Could you check a few things on this model? Use its own coordinates, in mm. A direction names the side the tool comes from. Give positions to 0.01 mm unless a question says otherwise; leave off trailing zeros. Loops run counter-clockwise (first coordinate to the right, second up) from the corner with the lowest first, then second, coordinate; pieces in that order, holes last. Notation, with made-up numbers: M 50,74.5 L 92,74.5 A18 ccw 92,91.5 Z; hole C 45.25,-38.75 d8. An arc over 180 degrees is marked long. Use CSV: the item, a comma, the result in double quotes.
```python
from build123d import *

# Parameters (mm, degrees)
SKETCH3_R           = 3.3
SKETCH3_R_2         = 2.3
BOSS_EXTRUDE3_DEPTH = 7
SKETCH4_R           = 5
SKETCH4_R_2         = 3.3
BOSS_EXTRUDE4_DEPTH = 2
SKETCH5_R           = 2.3
SKETCH5_R_2         = 1.7
BOSS_EXTRUDE5_DEPTH = 1


with BuildPart() as part:
    # Sketch3 → Boss-Extrude3 (new body)
    with BuildSketch(Plane(origin=(0, 0, 0), x_dir=(1, 0, 0), z_dir=(0, 1, 0))):
        Circle(SKETCH3_R)
        Circle(SKETCH3_R_2, mode=Mode.SUBTRACT)
    extrude(amount=BOSS_EXTRUDE3_DEPTH)

    # Sketch4 → Boss-Extrude4 (add)
    with BuildSketch(Plane.XZ):
        Circle(SKETCH4_R)
        Circle(SKETCH4_R_2, mode=Mode.SUBTRACT)
    extrude(amount=-BOSS_EXTRUDE4_DEPTH)

    # Sketch5 → Boss-Extrude5 (add)
    with BuildSketch(Plane(origin=(0, 7, 0), x_dir=(1, 0, 0), z_dir=(0, 1, 0))):
        Circle(SKETCH5_R)
        Circle(SKETCH5_R_2, mode=Mode.SUBTRACT)
    extrude(amount=-BOSS_EXTRUDE5_DEPTH)


solid = part.part
```
1. I'm going to push flat-ended pins straight in: pin 1 Ø4 at (y, z) = (1.5, 4) entering from -X; pin 2 Ø2 at (x, y) = (-3, 2.5) entering from -Z; pin 3 Ø1 at (x, y) = (-0.5, 3) entering from -Z. Where does each tip first touch, or does it pass through?
Outcome:
pin 1,"x = -4.58"
pin 2,"z = -4.52"
pin 3,"z = -3.3"
2. I want a section at D-D, the plane x = -4. List the corners of the cut face in (y, z) for me, then the cut area to 3 significant figures.
Outcome:
outline,"M 0,-3 L 2,-3 L 2,3 L 0,3 Z"
area,"12.0 mm2"
3. Which directions (+Z, -Z, +X, -X, +Y, -Y) give clear straight access to the entire face, cutting with the end or side of a thin tool? Please do faces 1 (the face through (-1.08, 0.99, -4.88)), 2 (the face through (-1.825, 2.958, 1.4)).
Outcome:
face 1,"+Y, -Y"
face 2,"-Y"
4. I want a section at C-C, the plane y = 4. List the corners of the cut face in (x, z) for me, then the cut area to 3 significant figures.
Outcome:
outline,"C 0,0 d6.6; hole C 0,0 d4.6"
area,"17.6 mm2"
5. Please list where these lines run through material, in increasing order: line 1 (X direction, y = 6.6, z = 0); line 2 (X direction, y = 3, z = 0).
Outcome:
line 1,"-3.3 to -1.7, 1.7 to 3.3"
line 2,"-3.3 to -2.3, 2.3 to 3.3"
6. If we mould it in two halves opening along Z, with no side actions, what happens to faces 3 (the face through (-0.37, 6.51, 1.66)), 4 (the face through (-2.43, 4.46, -2.23)), 5 (the face through (-1.2, 2, -3.3))? For each: +Z half, -Z half, draft (parallel to the pull), parting line (faces both ways), or undercut.
Outcome:
face 3,"undercut"
face 4,"parting line"
face 5,"draft"
7. I want a section at B-B, the plane x = -1.5. List the corners of the cut face in (y, z) for me, then the cut area to 4 significant figures.
Outcome:
outline,"M 0,-4.77 L 2,-4.77 L 2,-2.94 L 7,-2.94 L 7,-0.8 L 6,-0.8 L 6,-1.74 L 0,-1.74 Z; M 0,1.74 L 6,1.74 L 6,0.8 L 7,0.8 L 7,2.94 L 2,2.94 L 2,4.77 L 0,4.77 Z"
area,"25.95 mm2"
8. I want a section at A-A, the plane z = -0.5. List the corners of the cut face in (x, y) for me (3 decimals), then the cut area to 3 significant figures.
Outcome:
outline,"M -4.975,0 L -2.245,0 L -2.245,6 L -1.625,6 L -1.625,7 L -3.262,7 L -3.262,2 L -4.975,2 Z; M 1.625,6 L 2.245,6 L 2.245,0 L 4.975,0 L 4.975,2 L 3.262,2 L 3.262,7 L 1.625,7 Z"
area,"22.3 mm2"
